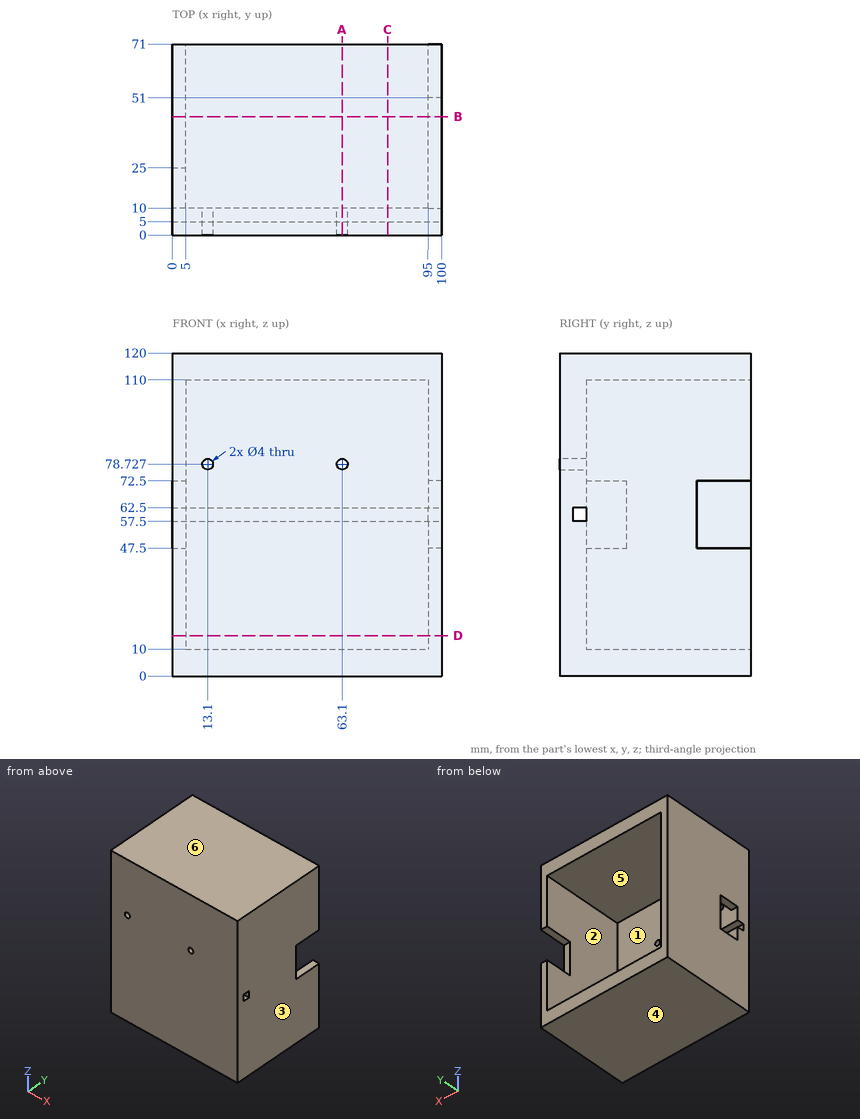
Study the drawing (mm; zero at the part's minimum x, y, z) and answer. A direction names the side the tool comes from. Give positions to 0.01 mm unless a question says otherwise; leave off trailing zeros. Loops run counter-clockwise (first coordinate to the right, second up) from the corner with the lowest first, then second, coordinate; pieces in that order, holes last. Notation, with made-up numbers: (88.5, 62.5) - (123.5, 62.5) arc R14 cw to (123.5, 73.5) - close; hole circle Ø7 at (-33.5, -0.5). An arc over 180 degrees is marked (long way). Answer as CSV lines item,"result". Start each with the question number.
1) Find section A-A (x = 63.1). Write down the section's boundary in (y, z).
2) Determine the mould class of the marked faces 1, 2, 3 and 4 for opening direction X: released by +X, released by -X, zero draft, split by the parting line, or undercut.
3) Each of these flat-tipped pins is pushed along its axis until it touches: pin 1 Ø2 at (x, z) = (90, 40) entering from +Y; pin 2 Ø2.5 at (x, z) = (68, 61) entering from +Y; pin 3 Ø1.5 at (x, z) = (98, 66) entering from +Y. Where does it stop, or does it pass through?
4) Which of the six approach directions +Z, -Z, +X, -X, +Y, -Y give full straight-line access (tool end or side, diameter ignored) to the marked faces 5 and 6?
5) Straight lines are drawn through the part: L1, parallel to Z at x = 13, y = 6; L2, parallel to Z at x = 26, y = 45; L3, parallel to Z at x = 63, y = 4. For each, find the intervals that lie inside material, in ascending order. Write a range as from..to.
6) Find section B-B (y = 44). Write down the section's boundary in (x, z).
7) Find section C-C (x = 80). Write down the section's boundary in (y, z).
8) Find section D-D (z = 15). Write down the section's boundary in (x, y).
Findings below:
1,outline,"(0, 0) - (71, 0) - (71, 10) - (10, 10) - (10, 57.5) - (5, 57.5) - (5, 62.5) - (10, 62.5) - (10, 76.73) - (0, 76.73) - close; (0, 80.73) - (10, 80.73) - (10, 110) - (71, 110) - (71, 120) - (0, 120) - close"
2,face 1,"undercut"
2,face 2,"undercut"
2,face 3,"released by +X"
2,face 4,"zero draft"
3,pin 1,"y = 10"
3,pin 2,"y = 5"
3,pin 3,"y = 51"
4,face 5,"+Y"
4,face 6,"+Z, +X, -X, +Y, -Y"
5,L1,"0..57.5, 62.5..76.73, 80.72..120"
5,L2,"0..10, 110..120"
5,L3,"0..76.73, 80.72..120"
6,outline,"(0, 0) - (100, 0) - (100, 120) - (0, 120) - close; hole (5, 10) - (95, 10) - (95, 110) - (5, 110) - close"
7,outline,"(0, 0) - (71, 0) - (71, 10) - (10, 10) - (10, 57.5) - (5, 57.5) - (5, 62.5) - (10, 62.5) - (10, 110) - (71, 110) - (71, 120) - (0, 120) - close"
8,outline,"(0, 0) - (100, 0) - (100, 71) - (95, 71) - (95, 10) - (5, 10) - (5, 71) - (0, 71) - close"
